Here's how the part is built. I have some questions about the finished solid (model axes, mm). Coordinates: 2 decimals unless noted, no trailing zeros. Write each loop counter-clockwise with the first axis right and the second up, starting at its lowest first coordinate (ties: lowest second). Pieces come first, ordered by that corner, then holes. Notation, with made-up numbers: (57, 26.5) -> (72, 26.5) arc R25 cw to (72, 47.5) -> close; hole circle Ø5 at (1, 67). An arc over 180 degrees is marked (long way). Put each result on its own line as item: value. Start each with the question number.
Item 1: If we mould it in two halves opening along Y, with no side actions, what happens to faces 1 (the face through (-2.539, -1.947, 0.789)), 2 (the face through (0, -14.432, 1)), 3 (the face through (-4, 1, 0))? For each: released by +Y, released by -Y, zero draft, split by the parting line, or undercut.
Item 2: I want a section at C-C, the plane z = 0.3. List the corners of the cut face in (x, y) for me.
Item 3: I want a section at B-B, the plane y = 0. List the corners of the cut face in (x, z) for me, then the cut area to 3 significant figures.
Item 4: I need wall thicknesses on line 1 (X direction, y = -8, z = 0.35); line 2 (Y direction, x = 7.5, z = 0.3); line 3 (Y direction, x = -6, z = 0.3). Which ranges of each line are inside material? Lowest first, please. Write a range as [from, to].
Item 5: I want a section at A-A, the plane x = 0. List the corners of the cut face in (y, z) for me, then the cut area to 3 significant figures.
from build123d import *

# Parameters (mm, degrees)
F0_R     = 1.6
F0_R_2   = 3.2
F1_DEPTH = 1.6


with BuildPart() as f1:
    # F0 (on Top) → F1 (new body)
    with BuildSketch(Plane.XY):
        with BuildLine():
            Line((-5.08, -14.432034), (5.08, -14.432034))
            ThreePointArc((5.08, -14.432034), (0, 15.3), (-5.08, -14.432034))
        make_face()
        with Locations((-6.717514, -6.717514)):
            Circle(F0_R, mode=Mode.SUBTRACT)
        with Locations((8.838835, -8.838835)):
            Circle(F0_R, mode=Mode.SUBTRACT)
        with Locations((5.656854, -5.656854)):
            Circle(F0_R, mode=Mode.SUBTRACT)
        Circle(F0_R_2, mode=Mode.SUBTRACT)
        with Locations((-5.656854, 5.656854)):
            Circle(F0_R, mode=Mode.SUBTRACT)
        with Locations((-8.838835, 8.838835)):
            Circle(F0_R, mode=Mode.SUBTRACT)
        with Locations((6.717514, 6.717514)):
            Circle(F0_R, mode=Mode.SUBTRACT)
    extrude(amount=F1_DEPTH)


solid = f1.part
Calculated:
1. face 1: undercut
1. face 2: released by -Y
1. face 3: zero draft
2. outline: (-5.08, -14.43) -> (5.08, -14.43) arc R15.3 ccw (long way) to start; hole circle Ø3.2 at (-8.84, 8.84); hole circle Ø3.2 at (-6.72, -6.72); hole circle Ø3.2 at (-5.66, 5.66); hole circle Ø6.4 at (0, 0); hole circle Ø3.2 at (5.66, -5.66); hole circle Ø3.2 at (6.72, 6.72); hole circle Ø3.2 at (8.84, -8.84)
3. outline: (-15.3, 0) -> (-3.2, 0) -> (-3.2, 1.6) -> (-15.3, 1.6) -> close; (3.2, 0) -> (15.3, 0) -> (15.3, 1.6) -> (3.2, 1.6) -> close
3. area: 38.7 mm2
4. line 1: x = [-13.04, -7.67], [-5.76, 7.48], [10.2, 13.04]
4. line 2: y = [-13.34, -9.71], [-7.96, 5.32], [8.11, 13.34]
4. line 3: y = [-14.07, -8.15], [-5.29, 4.09], [7.22, 14.07]
5. outline: (-14.43, 0) -> (-3.2, 0) -> (-3.2, 1.6) -> (-14.43, 1.6) -> close; (3.2, 0) -> (15.3, 0) -> (15.3, 1.6) -> (3.2, 1.6) -> close
5. area: 37.3 mm2
